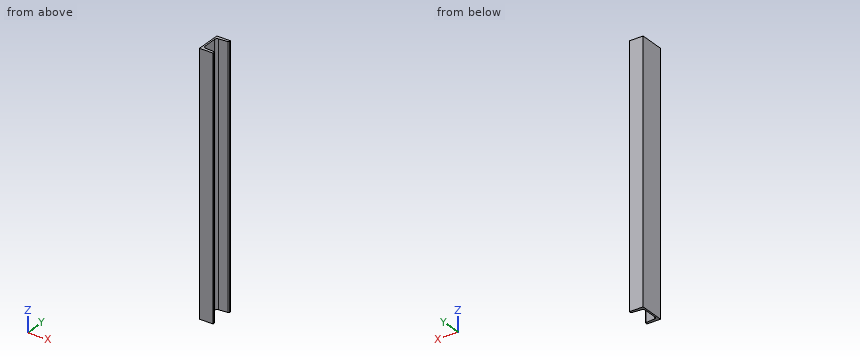
Autodesk Inventor part; units mm, degrees
ref_plane "Начальная плоскость" through (0, 0, 0) normal (0, 0, 1) x (1, 0, 0)
ref_plane "Конечная плоскость" through (0, 0, 667) normal (0, 0, 1) x (1, 0, 0)
ref_plane "YZ Plane" through (0, 0, 0) normal (1, 0, 0) x (0, 1, 0)
ref_plane "Начальная плоскость" through (0, 0, 0) normal (0, 0, 1) x (1, 0, 0)
ref_plane "Конечная плоскость" through (0, 0, 667) normal (0, 0, 1) x (1, 0, 0)
sketch "Эскиз" plane through (0, 0, 0) normal (0, 0, 1) x (1, 0, 0)
  line L0 (36, -32.5) -> (0, -32.5)
  line L1 (36, -32.5) -> (36, -28.696)
  line L2 (33.6994, -26.2039) -> (9.9215, -24.3017)
  line L3 (4.4, -18.3208) -> (4.4, 18.3208)
  line L4 (33.6994, 26.2039) -> (9.9215, 24.3017)
  line L5 (36, 28.696) -> (36, 32.5)
  line L6 (0, 32.5) -> (36, 32.5)
  line L7 (0, -32.5) -> (0, 32.5)
  arc A0 (4.4, -18.3208) -> (9.9215, -24.3017) centre (10.4, -18.3208) ccw
  arc A1 (9.9215, 24.3017) -> (4.4, 18.3208) centre (10.4, 18.3208) ccw
  arc A2 (36, -28.696) -> (33.6994, -26.2039) centre (33.5, -28.696) ccw
  arc A3 (33.6994, 26.2039) -> (36, 28.696) centre (33.5, 28.696) ccw
  line L8 (0, 45.5) -> (0, -45.5) construction
  line L9 (-7.2974, 0) -> (43.7847, 0) construction
  point P0 (36, -26.388)
  point P1 (4.4, -23.86)
  point P2 (4.4, 23.86)
  point P3 (36, 26.388)
  dimension "d3" = 36
  dimension "d5" = 4.4
  dimension "d7" = 65
  dimension "d9" = 8.64
  dimension "d11" = 8.64
  dimension "d13" = 6.112
  dimension "d15" = 6.112
  dimension "d22" = 6
  dimension "d23" = 2.5
  dimension "d24" = 32.5
  dimension "d25" = 0
extrude "Тело" add sketch "Эскиз" along normal up to surface (667 mm away) from surface at 0
sketch "Sketch3" plane through (0, 0, 0) normal (0, 0, 1) x (1, 0, 0)
  line L0 (0, 0) -> (10, 0)
ref_plane "Work Plane7" through (0, 0, 0) normal (0, -1, 0) x (1, 0, 0)
sketch "Sketch4" plane through (0, 0, 0) normal (0, -1, 0) x (1, 0, 0)
  line L0 (-2, 0) -> (12, 0)
  line L1 (-2, 667) -> (12, 667)
  dimension "d29" = 667
equation "\"d3\" = b"
equation "\"d7\" = ParH"
equation "\"d22\" = R"
equation "\"d23\" = R1"
equation "\"d24\" = 0.5 * d7"
equation "\"d16\" = G_L"
equation "\"R1\" = 2.5"
equation "\"R\" = 6"
equation "\"t1\" = 4.4"
equation "\"t2\" = 7.2"
equation "\"ParH\" = 65"
equation "\"b\" = 36"
equation "\"msp_x1\" = 0.04 * b"
equation "\"msp_x2\" = -0.08 * t1 + 0.04 * b"
equation "\"G_L\" = d29"
equation "\"ex\" = 0"
equation "\"G_OFFSET_START\" = 0"
equation "\"G_OFFSET_END\" = 0"
equation "\"d27\" = G_OFFSET_END + B_L"
equation "\"B_L\" = 667"
properties part number "Швеллер 6.5U-667 ГОСТ 8240-97" material "Сталь, мягкая"
Read the model definition and answer for the solid it produces. Units are mm, in the model's axes. Coordinates: 2 decimals unless noted, no trailing zeros. Write each loop counter-clockwise with the first axis right and the second up, starting at its lowest first coordinate (ties: lowest second). Pieces come first, ordered by that corner, then holes. Notation, with made-up numbers: (16.5, 16) -> (23.5, 16) arc R8 cw to (23.5, 23) -> close; hole circle Ø10 at (4.25, 47.5). An arc over 180 degrees is marked (long way). Return JSON: item names as keys, results as strings.
1. Find the intervals of material crossed by line 1 along Y through (x, z) = (34, 523.5); line 2 along X through (y, z) = (15, 608); line 3 along Y through (x, z) = (8, 50), in increasing order. Write a range as from..to.
Found:
{"line 1": "-32.5..-26.25, 26.25..32.5", "line 2": "0..4.4", "line 3": "-32.5..-23.82, 23.82..32.5"}
2. A cutting plane is placed at A-A (z = 332.5). Determine the outline of the cut face in (x, y).
Found:
{"outline": "(0, -32.5) -> (36, -32.5) -> (36, -28.7) arc R2.5 ccw to (33.7, -26.2) -> (9.92, -24.3) arc R6 cw to (4.4, -18.32) -> (4.4, 18.32) arc R6 cw to (9.92, 24.3) -> (33.7, 26.2) arc R2.5 ccw to (36, 28.7) -> (36, 32.5) -> (0, 32.5) -> close"}
3. A cutting plane is placed at C-C (y = 5). Determine the outline of the cut face in (x, z).
Found:
{"outline": "(0, 0) -> (4.4, 0) -> (4.4, 667) -> (0, 667) -> close"}
4. A cutting plane is placed at B-B (x = 19.5). Determine the outline of the cut face in (y, z).
Found:
{"outline": "(-32.5, 0) -> (-25.07, 0) -> (-25.07, 667) -> (-32.5, 667) -> close; (25.07, 0) -> (32.5, 0) -> (32.5, 667) -> (25.07, 667) -> close"}
5. Each of these flat-tipped pins is pushed along its axis until it touches: P1, Ø11, axis at y = -8, z = 212.5, coming from the +X side; P2, Ø8, axis at x = 9.5, y = -2.5, coming from the +Z side. Where does it stop, or does it pass through?
Found:
{"P1": "x = 4.4", "P2": "through"}
